from build123d import *


with BuildPart() as f2:
    # F0 (on Front) → F2 (revolve)
    with BuildSketch(Plane.XZ):
        with BuildLine():
            Line((-10, 2.5), (-3.5, 2.5))
            Line((-3.5, 2.5), (-2.5, 2.5))
            Line((-2.5, 2.5), (-2.5, 2))
            Line((-2.5, 2), (-1.5, 2))
            Line((-1.5, 2), (-1.5, 0.75))
            Line((-1.5, 0.75), (0, 0.75))
            Line((0, 0.75), (0, 3.5))
            ThreePointArc((0, 3.5), (-4.417261, 3.744651), (-8.780488, 4.47561))
            ThreePointArc((-8.780488, 4.47561), (-9.624695, 4.280869), (-10, 3.5))
            Line((-10, 3.5), (-10, 2.5))
        make_face()
    revolve(axis=Axis((0, 0, 5.189829), (0, 0, 1)))


solid = f2.part
Read the model definition and answer for the solid it produces. Units are mm, in the model's axes. A direction names the side the tool comes from. Coordinates: 2 decimals unless noted, no trailing zeros. Write each loop counter-clockwise with the first axis right and the second up, starting at its lowest first coordinate (ties: lowest second). Pieces come first, ordered by that corner, then holes. Notation, with made-up numbers: (23, -39) -> (35, -39) arc R4 cw to (35, -34) -> close; hole circle Ø11 at (6.5, -30.75). An arc over 180 degrees is marked (long way). Return JSON: item names as keys, results as strings.
(1) The part is cut by section A-A on z = 1.1. Give the vertices of the cut face in (x, y).
Answers below:
{"outline": "circle Ø3 at (0, 0)"}
(2) Consider line 1 along X through (y, z) = (-2, 2.1); line 2 along Z through (x, y) = (7.5, 5); line 3 along Z through (x, y) = (7.5, 5.75). Determine where each line is inside the solid, lowest interval first. Write a range as from..to.
Answers below:
{"line 1": "-1.5..1.5", "line 2": "2.5..4.5", "line 3": "2.5..4.39"}
(3) Which of the six approach directions +Z, -Z, +X, -X, +Y, -Y give full straight-line access (tool end or side, diameter ignored) to faces 1 (the flat face through (0, 0, 0.75)), 2 (the cylindrical face through (1.5, -0.07, 1.37))?
Answers below:
{"face 1": "-Z, +X, -X, +Y, -Y", "face 2": "-Z"}
(4) The part is cut by section B-B on z = 3.1. Give the vertices of the cut face in (x, y).
Answers below:
{"outline": "circle Ø20 at (0, 0)"}
(5) Each of these flat-tipped pins is pushed along its axis until it touches: P1, Ø3, axis at x = 7, y = 4.5, coming from the +Z side; P2, Ø6, axis at x = 3, y = 3.5, coming from the -Z side; P3, Ø1, axis at y = 2, z = 2.5, coming from the +X side; P4, Ø2, axis at y = 5, z = 4, coming from the +X side. Where does it stop, or does it pass through?
Answers below:
{"P1": "z = 4.5", "P2": "z = 2", "P3": "x = 9.89", "P4": "x = 9.12"}
